from build123d import *

# Parameters (mm, degrees)
SKETCH1_W               = 271.78
SKETCH1_H               = 152.4
BOSS_EXTRUDE1_DEPTH     = 6.35
SKETCH2_W               = 6.35
SKETCH2_H               = 19.05
CUT_EXTRUDE1_DEPTH      = 156.925798379
LPATTERN1_COUNT         = 4
LPATTERN1_PITCH         = 38.1
MIRROR1_COPY_1_SKETCH_W = 6.35
MIRROR1_COPY_1_SKETCH_H = 19.05
MIRROR1_COPY_1_DEPTH    = 156.925798379
MIRROR1_COPY_2_SKETCH_W = 6.35
MIRROR1_COPY_2_SKETCH_H = 19.05
MIRROR1_COPY_2_DEPTH    = 156.925798379
MIRROR1_COPY_3_SKETCH_W = 6.35
MIRROR1_COPY_3_SKETCH_H = 19.05
MIRROR1_COPY_3_DEPTH    = 156.925798379


with BuildPart() as part:
    # Sketch1 → Boss-Extrude1 (new body)
    with BuildSketch(Plane.XY):
        Rectangle(SKETCH1_W, SKETCH1_H)
    extrude(amount=BOSS_EXTRUDE1_DEPTH)

    # Sketch2 → Cut-Extrude1 (cut, through all)
    with BuildSketch(Plane.XY.offset(6.35)):
        with Locations((-132.715, 60.325)):
            Rectangle(SKETCH2_W, SKETCH2_H)
    cut_extrude1 = extrude(amount=-CUT_EXTRUDE1_DEPTH, mode=Mode.SUBTRACT)

    # LPattern1: Cut-Extrude1 ×4
    with Locations(*[(0, -i * LPATTERN1_PITCH, 0) for i in range(1, LPATTERN1_COUNT)]):
        add(cut_extrude1, mode=Mode.SUBTRACT)

    # Mirror1: Cut-Extrude1 across plane
    add(cut_extrude1.mirror(Plane(origin=(0, 0, 0), x_dir=(0, 0, 1), z_dir=(1, 0, 0))), mode=Mode.SUBTRACT)

    # Mirror1 copy 1 sketch → Mirror1 copy 1 (cut, through all)
    with BuildSketch(Plane(origin=(0, -38.1, 6.35), x_dir=(-1, 0, 0), z_dir=(0, 0, 1))):
        with Locations((-132.715, -60.325)):
            Rectangle(MIRROR1_COPY_1_SKETCH_W, MIRROR1_COPY_1_SKETCH_H)
    extrude(amount=-MIRROR1_COPY_1_DEPTH, mode=Mode.SUBTRACT)

    # Mirror1 copy 2 sketch → Mirror1 copy 2 (cut, through all)
    with BuildSketch(Plane(origin=(0, -76.2, 6.35), x_dir=(-1, 0, 0), z_dir=(0, 0, 1))):
        with Locations((-132.715, -60.325)):
            Rectangle(MIRROR1_COPY_2_SKETCH_W, MIRROR1_COPY_2_SKETCH_H)
    extrude(amount=-MIRROR1_COPY_2_DEPTH, mode=Mode.SUBTRACT)

    # Mirror1 copy 3 sketch → Mirror1 copy 3 (cut, through all)
    with BuildSketch(Plane(origin=(0, -114.3, 6.35), x_dir=(-1, 0, 0), z_dir=(0, 0, 1))):
        with Locations((-132.715, -60.325)):
            Rectangle(MIRROR1_COPY_3_SKETCH_W, MIRROR1_COPY_3_SKETCH_H)
    extrude(amount=-MIRROR1_COPY_3_DEPTH, mode=Mode.SUBTRACT)


solid = part.part
Design review of the part built by this model. Coordinates are the model's own, in mm. A direction names the side the tool comes from. Round coordinates to 2 decimals unless told otherwise and drop trailing zeros. Order: outer loops, then holes, each group sorted by start corner. A loop starts at its lowest first (then second) coordinate and runs counter-clockwise, first axis right, second up.
1) For L1, parallel to X at y = 31, z = 2.5, list the stretches that pass through material, from the lowest coordinate up.
The answers:
L1: x = -129.54 to 129.54
2) Draft analysis for pull direction Y (two halves, no side actions). For faces 4 (the flat face through (-133, 50.8, 3)), 5 (the flat face through (-2, 1, 0)), state which applies: released by +Y, released by -Y, zero draft, split by the parting line, or undercut.
The answers:
face 4: undercut
face 5: zero draft
3) Machinability: for faces 1 (the flat face through (-133, -63.5, 3)), 2 (the flat face through (133, -44.45, 3)), 3 (the flat face through (-135.89, -35, 3)), which of the approach directions +Z, -Z, +X, -X, +Y, -Y give a long, thin tool a straight path to every point of the face, cutting with its end or side? Answer none if there is none.
The answers:
face 1: +Z, -Z, -X
face 2: +Z, -Z, +X
face 3: +Z, -Z, -X, +Y, -Y
4) Clearance check with flat-ended pins moving along their axes: pin 1 Ø3 at (y, z) = (-61, 5) entering from -X; pin 2 Ø1.9 at (y, z) = (-53, 2.5) entering from +X. State where each tip first meets the part, or that it passes through.
The answers:
pin 1: stops at x = -129.54
pin 2: stops at x = 129.54
5) Consider section A-A (y = -61). State the section outline as (x, z) points.
The answers:
outline: (-129.54, 0) - (129.54, 0) - (129.54, 6.35) - (-129.54, 6.35) - close
